Geometry: final body of the model. Coordinates: model frame, mm. Give positions to 0.01 mm unless a question says otherwise; leave off trailing zeros. Write each loop counter-clockwise with the first axis right and the second up, starting at its lowest first coordinate (ties: lowest second). Pieces come first, ordered by that corner, then holes. Notation, with made-up numbers: (-9.75, 15) -> (25.25, 15) arc R19 ccw to (25.25, 33) -> close; hole circle Ø5 at (78, -6). An arc over 180 degrees is marked (long way). Answer as a JSON object with one key per item and string values.
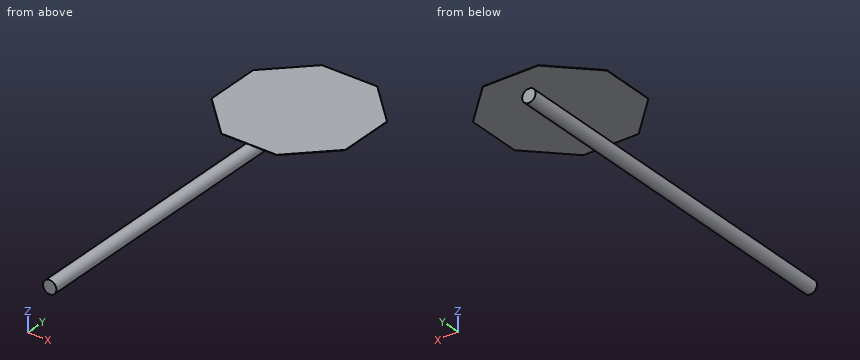
from build123d import *

# Parameters (mm, degrees)
SKETCH3_R           = 38.1
BOSS_EXTRUDE1_DEPTH = 2133.6
BOSS_EXTRUDE2_START = 38.1
BOSS_EXTRUDE2_DEPTH = 1.016


with BuildPart() as part:
    # Sketch3 → Boss-Extrude1 (new body)
    with BuildSketch(Plane(origin=(0, 0, 0), x_dir=(1, 0, 0), z_dir=(0, 1, 0))):
        with Locations(Location((0, 0, 0), (0, 0, 270))):
            Circle(SKETCH3_R)
    extrude(amount=BOSS_EXTRUDE1_DEPTH)

    # Sketch5 → Boss-Extrude2 (add, symmetric)
    with BuildSketch(Plane.XY.offset(BOSS_EXTRUDE2_START)):
        Polygon((-381, 1734.484632736), (-157.815367264, 1511.3), (157.815367264, 1511.3), (381, 1734.484632736), (381, 2050.115367264), (157.815367264, 2273.3), (-157.815367264, 2273.3), (-381, 2050.115367264), align=None)
    extrude(amount=BOSS_EXTRUDE2_DEPTH, both=True)


solid = part.part
Q1. Cut plane D-D (y = 432). Return the cut outline in (x, z), and give its area (3 significant figures).
Values:
{"outline": "circle Ø76.2 at (0, 0)", "area": "4,560 mm²"}
Q2. Material intervals for L1, parallel to Z at x = -113, y = 1774; L2, parallel to Y at x = -6, z = 28.5; L3, parallel to X at y = 1125, z = 2, sorted ascending. Write a range as from..to.
Values:
{"L1": "37.08..39.12", "L2": "0..2133.6", "L3": "-38.05..38.05"}
Q3. First-contact query: P1, Ø2, axis at y = 699, z = -6.5, coming from the +X side; P2, Ø8, axis at y = 1320.5, z = 30.5, coming from the -X side; P3, Ø3, axis at y = 646, z = -27, coming from the +X side; P4, Ø12, axis at x = 47.5, y = 800.5, coming from the +Z side. Flat tips, straight axial feed; report the tip coordinate or a pass-through.
Values:
{"P1": "x = 37.7", "P2": "x = -27.37", "P3": "x = 28.31", "P4": "through"}
Q4. Cut plane C-C (x = -137). Return the cut outline in (y, z).
Values:
{"outline": "(1511.3, 37.08) -> (2273.3, 37.08) -> (2273.3, 39.12) -> (1511.3, 39.12) -> close"}
Q5. Cut plane A-A (y = 1595). Return the cut outline in (x, z), and give its area (3 significant figures).
Values:
{"outline": "(-241.52, 37.08) -> (-8.74, 37.08) arc R38.1 ccw (long way) to (8.74, 37.08) -> (241.52, 37.08) -> (241.52, 39.12) -> (-241.52, 39.12) -> close", "area": "5,530 mm²"}
Q6. Cut plane B-B (z = 0). Return the cut outline in (x, y), and give its area (3 significant figures).
Values:
{"outline": "(-38.1, 0) -> (38.1, 0) -> (38.1, 2133.6) -> (-38.1, 2133.6) -> close", "area": "163,000 mm²"}
